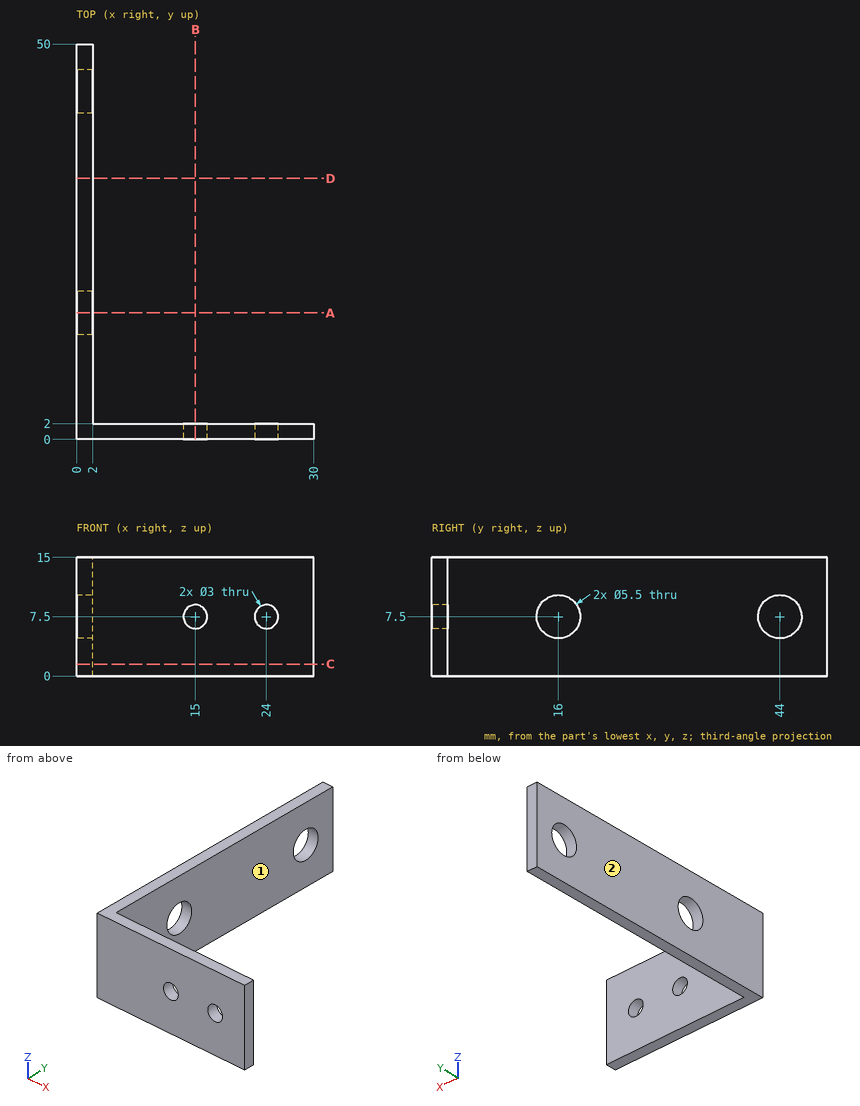
The drawing under review shows one solid part. Ordinate dimensions are in mm from its lowest x, y, z. A direction names the side the tool comes from. Coordinates: 2 decimals unless noted, no trailing zeros. Write each loop counter-clockwise with the first axis right and the second up, starting at its lowest first coordinate (ties: lowest second). Pieces come first, ordered by that corner, then holes. Notation, with made-up numbers: (6.25, 86.25) - (52.25, 86.25) arc R3 cw to (52.25, 90.25) - close; hole circle Ø6 at (66, 69.25). An arc over 180 degrees is marked (long way). Use one line per item in the form item = value.
Q1. Machinability: for the marked faces 1 and 2, which of the approach directions +Z, -Z, +X, -X, +Y, -Y give a long, thin tool a straight path to every point of the face, cutting with its end or side? Answer none if there is none.
Taken from the geometry:
face_1 = +Z, -Z, +X, +Y
face_2 = +Z, -Z, -X, +Y, -Y
Q2. Consider section A-A (y = 16). Write out the cut boundary in (x, z), plus the area to 3 significant figures.
Taken from the geometry:
outline = (0, 0) - (2, 0) - (2, 4.75) - (0, 4.75) - close; (0, 10.25) - (2, 10.25) - (2, 15) - (0, 15) - close
area = 19.0 mm^2
Q3. Consider section B-B (x = 15). Write out the cut boundary in (y, z), plus the area to 3 significant figures.
Taken from the geometry:
outline = (0, 0) - (2, 0) - (2, 6) - (0, 6) - close; (0, 9) - (2, 9) - (2, 15) - (0, 15) - close
area = 24.0 mm^2
Q4. For probe 1 along Y at (x, z) = (1.6, 7.5); probe 2 along Y at (x, z) = (17.25, 8.25), list the stretches that pass through material, from the lowest coordinate up.
Taken from the geometry:
probe_1 = 0 to 13.25, 18.75 to 41.25, 46.75 to 50
probe_2 = 0 to 2
Q5. Insertion check: pin 1 Ø10 at (x, y) = (11, 12) entering from +Z; pin 2 Ø6 at (y, z) = (36.5, 3) entering from -X; pin 3 Ø7 at (y, z) = (44, 7.5) entering from +X; pin 4 Ø4.5 at (x, z) = (20, 8.5) entering from +Y. Each pin has a flat end and moves straight along its axis. Give the tip position at first contact, or say it passes through.
Taken from the geometry:
pin_1 = through
pin_2 = 0
pin_3 = 2
pin_4 = 2
Q6. Consider section C-C (z = 1.5). Write out the cut boundary in (x, y).
Taken from the geometry:
outline = (0, 0) - (30, 0) - (30, 2) - (2, 2) - (2, 50) - (0, 50) - close
Q7. Consider section D-D (y = 33). Write out the cut boundary in (x, z), plus the area to 3 significant figures.
Taken from the geometry:
outline = (0, 0) - (2, 0) - (2, 15) - (0, 15) - close
area = 30.0 mm^2
